from build123d import *

# Parameters (mm, degrees)
PAD014_DEPTH    = 5
THICKNESS001_T  = -2
SKETCH029_R     = 4.5
POCKET011_DEPTH = 5.001
SKETCH030_R     = 3
PAD015_DEPTH    = 3
SKETCH031_R     = 1.65
POCKET012_DEPTH = 3.3
POCKET_DEPTH    = 2
CHAMFER_SIZE    = 1
CHAMFER002_SIZE = 1.5


with BuildPart() as part:
    # Sketch027 → Pad014 (new body)
    with BuildSketch(Plane(origin=(0, 0, 0), x_dir=(-1, 0, 0), z_dir=(0, 0, 1))):
        with BuildLine():
            Line((-23.4, -44.000002), (-23.4, -1))
            ThreePointArc((-20, 2.4), (-22.404163, 1.404163), (-23.4, -1))
            Line((-20, 2.4), (-1, 2.4))
            ThreePointArc((2.4, -1), (1.404163, 1.404163), (-1, 2.4))
            Line((2.4, -1), (2.4, -44.000001))
            ThreePointArc((-0.999999, -47.4), (1.404163, -46.404163), (2.4, -44.000001))
            Line((-0.999999, -47.4), (-20.000001, -47.4))
            ThreePointArc((-23.4, -44.000002), (-22.404163, -46.404164), (-20.000001, -47.4))
        make_face()
    extrude(amount=PAD014_DEPTH)

    # Thickness001
    thickness001_openings = [part.faces().sort_by_distance(p)[0] for p in [
        (10.5, 22.5, 0),
    ]]
    offset(amount=THICKNESS001_T, openings=thickness001_openings)

    # Sketch029 (on Face9 of Thickness001) → Pocket011 (cut, through all)
    with BuildSketch(Plane.XY.offset(5)):
        with Locations((10.964466, 9.964466)):
            Circle(SKETCH029_R)
        with Locations((10.964466, 28.52028)):
            Circle(SKETCH029_R)
    extrude(amount=-POCKET011_DEPTH, mode=Mode.SUBTRACT)

    # Sketch030 (on Face4 of Pocket011) → Pad015 (join)
    with BuildSketch(Plane(origin=(0, 0, 0), x_dir=(1, 0, 0), z_dir=(0, 0, -1))):
        with Locations((3, -3)):
            Circle(SKETCH030_R)
        with Locations((18, -3)):
            Circle(SKETCH030_R)
        with Locations((18, -42)):
            Circle(SKETCH030_R)
        with Locations((3, -42)):
            Circle(SKETCH030_R)
    extrude(amount=-PAD015_DEPTH)

    # Sketch031 (on Face27 of Pad015) → Pocket012 (cut)
    with BuildSketch(Plane(origin=(0, 0, 0), x_dir=(1, 0, 0), z_dir=(0, 0, -1))):
        with Locations((3, -3)):
            Circle(SKETCH031_R)
        with Locations((18, -3)):
            Circle(SKETCH031_R)
        with Locations((18, -42)):
            Circle(SKETCH031_R)
        with Locations((3, -42)):
            Circle(SKETCH031_R)
    extrude(amount=-POCKET012_DEPTH, mode=Mode.SUBTRACT)

    # Sketch033 (on Face6 of Pocket012) → Pocket (cut)
    with BuildSketch(Plane(origin=(0, 47.4, 0), x_dir=(-1, 0, 0), z_dir=(0, 1, 0))):
        with BuildLine():
            Line((-14.661912, 0), (-7.262061, 0))
            Line((-7.262061, 0), (-7.262061, 1.787056))
            ThreePointArc((-7.262061, 1.787056), (-7.348276, 1.995197), (-7.556417, 2.081412))
            Line((-7.556417, 2.081412), (-14.367556, 2.081412))
            ThreePointArc((-14.367556, 2.081412), (-14.575697, 1.995197), (-14.661912, 1.787056))
            Line((-14.661912, 1.787056), (-14.661912, 0))
        make_face()
    extrude(amount=-POCKET_DEPTH, mode=Mode.SUBTRACT)

    # Chamfer
    chamfer_edges = [part.edges().sort_by_distance(p)[0] for p in [
        (6.464466, 28.52028, 5),
        (6.464466, 9.964466, 5),
    ]]
    chamfer(chamfer_edges, length=CHAMFER_SIZE)

    # Chamfer002
    chamfer002_edges = [part.edges().sort_by_distance(p)[0] for p in [
        (10.5, 47.4, 5),
    ]]
    chamfer(chamfer002_edges, length=CHAMFER002_SIZE)


solid = part.part
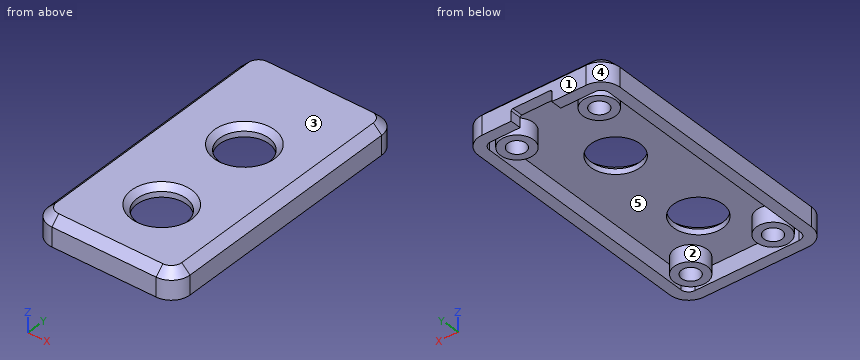
Can you work these out from the model? Positions are in its coordinate system, mm. Face numbers are marked on the shaded views. A direction names the side the tool comes from. Coordinates: 2 decimals unless noted, no trailing zeros. Write each loop counter-clockwise with the first axis right and the second up, starting at its lowest first coordinate (ties: lowest second). Pieces come first, ordered by that corner, then holes. Notation, with made-up numbers: (84, 76.5) -> (100, 76.5) arc R9 cw to (100, 93.5) -> close; hole circle Ø8 at (34, 4). An arc over 180 degrees is marked (long way). Write item = value, one per line.
(1) Imagine slicing it at C-C (x = 12.5). State how many separate pieces and enclosed holes the cut face has, and give its area (3 significant figures).
Verdict:
separate_pieces = 3
enclosed_holes = 0
area = 69.2 mm^2
(2) Imagine slicing it at B-B (x = 18). Please give me the cut outline in (y, z), and give its area (3 significant figures).
Verdict:
outline = (-2.4, 0) -> (-0.4, 0) -> (-0.4, 3) -> (0, 3) -> (0, 0) -> (1.35, 0) -> (1.35, 3.3) -> (4.65, 3.3) -> (4.65, 0) -> (6, 0) -> (6, 3) -> (39, 3) -> (39, 0) -> (40.35, 0) -> (40.35, 3.3) -> (43.65, 3.3) -> (43.65, 0) -> (45, 0) -> (45, 3) -> (45.4, 3) -> (45.4, 0) -> (47.4, 0) -> (47.4, 3.5) -> (45.9, 5) -> (-0.9, 5) -> (-2.4, 3.5) -> close
area = 124 mm^2
(3) For pin 1 (1 mm diameter, centred on x = 3.5, y = 3, fed in from -Z); pin 2 (0.9 mm diameter, centred on y = 46.5, z = 0.5, fed in from -X); pin 3 (5 mm diameter, centred on x = 6, y = 15.5, fed in from -Z); pin 4 (4.5 mm diameter, centred on x = 3, y = 3, fed in from -Z), each with a flat end and sliding along its axis, tell me the tip position at first contact or that it passes through.
Verdict:
pin_1 = 3.3
pin_2 = -1.71
pin_3 = 3
pin_4 = 0
(4) If I drill on probe 1 along Y at (x, z) = (3, 1.7); probe 2 along X at (y, z) = (36.5, 2.45); probe 3 along X at (y, z) = (42, 2.55), over which ranges is the centre line in solid material (lowest first)?
Verdict:
probe_1 = -2.4 to -0.4, 0 to 1.35, 4.65 to 6, 39 to 40.35, 43.65 to 45, 45.4 to 47.4
probe_2 = -2.4 to -0.4, 21.4 to 23.4
probe_3 = -2.4 to -0.4, 0 to 1.35, 4.65 to 6, 15 to 16.35, 19.65 to 21, 21.4 to 23.4
(5) Thinking about a two-plate mould opening in Y: for the marked faces 1, 2 and 3, which applies, +Y half, -Y half, draft (parallel to the pull), parting line (faces both ways), or undercut?
Verdict:
face_1 = +Y half
face_2 = undercut
face_3 = draft
(6) Imagine slicing it at A-A (y = 42). Please give me the cut outline in (x, z).
Verdict:
outline = (-2.4, 0) -> (-0.4, 0) -> (-0.4, 3) -> (0, 3) -> (0, 0) -> (1.35, 0) -> (1.35, 3.3) -> (4.65, 3.3) -> (4.65, 0) -> (6, 0) -> (6, 3) -> (15, 3) -> (15, 0) -> (16.35, 0) -> (16.35, 3.3) -> (19.65, 3.3) -> (19.65, 0) -> (21, 0) -> (21, 3) -> (21.4, 3) -> (21.4, 0) -> (23.4, 0) -> (23.4, 3.5) -> (21.9, 5) -> (-0.9, 5) -> (-2.4, 3.5) -> close
(7) On a 3-axis mill with a long thin cutter (end or side, diameter ignored), from which of +Z, -Z, +X, -X, +Y, -Y can I reach the whole of each face in a straight line? I mean the marked faces 4 and 5. Say none if no direction works.
Verdict:
face_4 = +Z, -Z, -X, +Y
face_5 = -Z
(8) Imagine slicing it at D-D (y = 18.5). Please give me the cut outline in (x, z), and give its area (4 significant figures).
Verdict:
outline = (-2.4, 0) -> (-0.4, 0) -> (-0.4, 3) -> (21.4, 3) -> (21.4, 0) -> (23.4, 0) -> (23.4, 3.5) -> (21.9, 5) -> (-0.9, 5) -> (-2.4, 3.5) -> close
area = 61.35 mm^2
